Input: part model. Units: mm. Frame: model coordinates. Round coordinates to 2 decimals unless told otherwise and drop trailing zeros. Order: outer loops, then holes, each group sorted by start corner. A loop starts at its lowest first (then second) coordinate and runs counter-clockwise, first axis right, second up. Notation, with made-up numbers: (84.25, 77.5) -> (109.25, 77.5) arc R25 ccw to (109.25, 99.5) -> close; hole circle Ø5 at (17, 84.5). An arc over 180 degrees is marked (long way). Use a Markdown table: item, result.
from build123d import *

# Parameters (mm, degrees)
F1_DEPTH = 8
F2_R     = 1.75
F3_DEPTH = 5
F4_R     = 1


with BuildPart() as f1:
    # F0 (on Top) → F1 (new body)
    with BuildSketch(Plane.XY):
        Polygon((4.049788, -3.174863), (4.049788, 1.825137), (-11.450212, 1.825137), (-11.450212, -1.174863), (-2.950212, -2.174863), (-2.950212, -3.174863), align=None)
    extrude(amount=F1_DEPTH)

    # F2 (on face) → F3 (cut, through all)
    with BuildSketch(Plane(origin=(0, 1.825137, 0), x_dir=(-1, 0, 0), z_dir=(0, 1, 0))):
        with Locations((-0.549788, 4)):
            Circle(F2_R)
    extrude(amount=-F3_DEPTH, mode=Mode.SUBTRACT)

    # F4
    f4_edges = [f1.edges().sort_by_distance(p)[0] for p in [
        (-11.450212, -1.174863, 4),
    ]]
    fillet(f4_edges, radius=F4_R)


solid = f1.part
1) Draft query along X for faces 1 (the face through (-2.95, -3, 4)), 2 (the face through (0.93, -0.64, 2.29)), 3 (the face through (4.05, -1, 4)). Return one class per face: released by +X, released by -X, zero draft, split by the parting line, or undercut.
Answer key:
| item | result |
|---|---|
| face 1 | released by -X |
| face 2 | undercut |
| face 3 | released by +X |
2) Cut plane A-A on z = 4. Return loops of the section in (x, y), and give its area (3 significant figures).
Answer key:
| item | result |
|---|---|
| outline | (-11.45, -0.29) arc R1 ccw to (-10.57, -1.28) -> (-2.95, -2.17) -> (-2.95, -3.17) -> (-1.2, -3.17) -> (-1.2, 1.83) -> (-11.45, 1.83) -> close; (2.3, -3.17) -> (4.05, -3.17) -> (4.05, 1.83) -> (2.3, 1.83) -> close |
| area | 47.1 mm^2 |
3) Ray query, probe 1 along Z at (x, y) = (0, 1.2); probe 2 along X at (y, z) = (0.8, 4.75); probe 3 along X at (y, z) = (1.1, 2.5). Return the intervals inside material, ascending.
Answer key:
| item | result |
|---|---|
| probe 1 | z = 0 to 2.34, 5.66 to 8 |
| probe 2 | x = -11.45 to -1.03, 2.13 to 4.05 |
| probe 3 | x = -11.45 to -0.35, 1.45 to 4.05 |
4) Cut plane B-B on x = -0.75. Return loops of the section in (y, z), and give its area (3 significant figures).
Answer key:
| item | result |
|---|---|
| outline | (-3.17, 0) -> (1.83, 0) -> (1.83, 2.83) -> (-3.17, 2.83) -> close; (-3.17, 5.17) -> (1.83, 5.17) -> (1.83, 8) -> (-3.17, 8) -> close |
| area | 28.3 mm^2 |
5) Cut plane D-D on y = 1.2. Return loops of the section in (x, z), and give its area (3 significant figures).
Answer key:
| item | result |
|---|---|
| outline | (-11.45, 0) -> (4.05, 0) -> (4.05, 8) -> (-11.45, 8) -> close; hole circle Ø3.5 at (0.55, 4) |
| area | 114 mm^2 |
6) Cut plane C-C on z = 1.5. Return loops of the section in (x, y), and give its area (3 significant figures).
Answer key:
| item | result |
|---|---|
| outline | (-11.45, -0.29) arc R1 ccw to (-10.57, -1.28) -> (-2.95, -2.17) -> (-2.95, -3.17) -> (4.05, -3.17) -> (4.05, 1.83) -> (-11.45, 1.83) -> close |
| area | 64.6 mm^2 |
